```python
from build123d import *

# Parameters (mm, degrees)
F1_DEPTH = 6.35
F2_W     = 6.35
F2_H     = 6.35
F3_DEPTH = 6.351


with BuildPart() as f1:
    # F0 (on Right) → F1 (new body)
    with BuildSketch(Plane.YZ):
        Polygon((-38.1, 38.1), (-44.45, 38.1), (-44.45, 31.75), (-50.8, 31.75), (-50.8, 25.4), (-44.45, 25.4), (-44.45, 19.05), (-50.8, 19.05), (-50.8, 12.7), (-44.45, 12.7), (-44.45, 6.35), (-50.8, 6.35), (-50.8, 0), (-50.8, -6.35), (-44.45, -6.35), (-44.45, -12.7), (-50.8, -12.7), (-50.8, -19.05), (-44.45, -19.05), (-44.45, -25.4), (-50.8, -25.4), (-50.8, -31.75), (-44.45, -31.75), (-44.45, -38.1), (-38.1, -38.1), (-38.1, -31.75), (-31.75, -31.75), (-31.75, -38.1), (-25.4, -38.1), (-25.4, -31.75), (-19.05, -31.75), (-19.05, -38.1), (-12.7, -38.1), (-12.7, -31.75), (-6.35, -31.75), (-6.35, -38.1), (0, -38.1), (6.35, -38.1), (6.35, -31.75), (12.7, -31.75), (12.7, -38.1), (19.05, -38.1), (19.05, -31.75), (25.4, -31.75), (25.4, -38.1), (31.75, -38.1), (31.75, -31.75), (38.1, -31.75), (38.1, -38.1), (44.45, -38.1), (44.45, -31.75), (50.8, -31.75), (50.8, -25.4), (44.45, -25.4), (44.45, -19.05), (50.8, -19.05), (50.8, -12.7), (44.45, -12.7), (44.45, -6.35), (50.8, -6.35), (50.8, 0), (50.8, 6.35), (44.45, 6.35), (44.45, 12.7), (50.8, 12.7), (50.8, 19.05), (44.45, 19.05), (44.45, 25.4), (50.8, 25.4), (50.8, 31.75), (44.45, 31.75), (44.45, 38.1), (38.1, 38.1), (38.1, 31.75), (31.75, 31.75), (31.75, 38.1), (25.4, 38.1), (25.4, 31.75), (19.05, 31.75), (19.05, 38.1), (12.7, 38.1), (12.7, 31.75), (6.35, 31.75), (6.35, 38.1), (0, 38.1), (-6.35, 38.1), (-6.35, 31.75), (-12.7, 31.75), (-12.7, 38.1), (-19.05, 38.1), (-19.05, 31.75), (-25.4, 31.75), (-25.4, 38.1), (-31.75, 38.1), (-31.75, 31.75), (-38.1, 31.75), align=None)
    extrude(amount=F1_DEPTH)

    # F2 (on face) → F3 (cut, through all)
    with BuildSketch(Plane.YZ.offset(6.35)):
        with BuildLine():
            ThreePointArc((-15.875, -6.35), (-12.7, -7.6651280605), (-9.525, -6.35))
            Line((-9.525, -6.35), (-15.875, -6.35))
        make_face()
        Polygon((-15.875, -6.35), (-9.525, -6.35), (-9.525, -3.175), (-9.525, 0), (-15.875, 0), align=None)
        with BuildLine():
            Line((-9.525, -3.175), (-9.525, -6.35))
            ThreePointArc((-9.525, -6.35), (-8.5516625865, -4.893297618), (-8.2098719395, -3.175))
            ThreePointArc((-8.2098719395, -3.175), (-8.5516625865, -1.456702382), (-9.525, 0))
            Line((-9.525, 0), (-9.525, -3.175))
        make_face()
        with BuildLine():
            ThreePointArc((-15.875, 0), (-17.1901280605, -3.175), (-15.875, -6.35))
            Line((-15.875, -6.35), (-15.875, 0))
        make_face()
        with BuildLine():
            Line((-15.875, 0), (-9.525, 0))
            ThreePointArc((-9.525, 0), (-12.7, 1.3151280605), (-15.875, 0))
        make_face()
        with BuildLine():
            ThreePointArc((22.225, 0), (19.05, 1.3151280605), (15.875, 0))
            Line((15.875, 0), (22.225, 0))
        make_face()
        with Locations((19.05, -3.175)):
            Rectangle(F2_W, F2_H)
        with BuildLine():
            Line((15.875, -6.35), (15.875, 0))
            ThreePointArc((15.875, 0), (14.5598719395, -3.175), (15.875, -6.35))
        make_face()
        with BuildLine():
            ThreePointArc((23.5401280605, -3.175), (23.1983374135, -1.456702382), (22.225, 0))
            Line((22.225, 0), (22.225, -6.35))
            ThreePointArc((22.225, -6.35), (23.1983374135, -4.893297618), (23.5401280605, -3.175))
        make_face()
        with BuildLine():
            Line((22.225, -6.35), (15.875, -6.35))
            ThreePointArc((15.875, -6.35), (19.05, -7.6651280605), (22.225, -6.35))
        make_face()
    extrude(amount=-F3_DEPTH, mode=Mode.SUBTRACT)


solid = f1.part
```
Part model, mm, in its own coordinate system. A direction names the side the tool comes from. Give positions to 0.01 mm unless a question says otherwise; leave off trailing zeros. Order: outer loops, then holes, each group sorted by start corner. A loop starts at its lowest first (then second) coordinate and runs counter-clockwise, first axis right, second up. Notation, with made-up numbers: M 39.25,43.25 L 48.25,43.25 A19 ccw 48.25,47.25 Z; hole C 34.25,-11 d6. An arc over 180 degrees is marked long. Use a Markdown table: item, result. Add a question column.
(1) Saw through at A-A, the plane y = 35. Give the cut face in (x, z), and give its area (3 significant figures).
(2) 3-axis set-ups, long thin cutter, end or side, ignore diameter. For faces 5 (the face through (3, -48, -19.05)), 6 (the face through (3, -31.75, 35)), 7 (the face through (3, 48, -31.75)), 8 (the face through (3, 31.75, -35)): which of +Z, -Z, +X, -X, +Y, -Y reach the whole face in a straight line?
(3) Probe line 1 along Z through (x, y) = (3.5, 45.5); line 2 along Z through (x, y) = (6, -13); line 3 along Y through (x, z) = (1.75, -11.5). List the from-to ranges inside material, lowest first. Write a range as [from, to].
(4) Saw through at B-B, the plane x = 2. Give the number of separate pieces and of enclosed holes in the cut face, and give its area (3 significant figures).
(5) Drop flat-ended pins along their axis: P1, Ø3, axis at x = 4, z = 34, coming from the +Y side; P2, Ø3, axis at x = 4.5, z = -34.5, coming from the -Y side; P3, Ø1.9, axis at x = 3.5, y = -49, coming from the -Z side; P4, Ø2, axis at x = 5, y = 7, coming from the -Z side. Give the stop position or say it passes through.
(6) Saw through at C-C, the plane z = -21.5. Give the cut face in (x, y), and give its area (3 significant figures).
(7) Mould opens along Y. For faces 1 (the face through (3, -50.8, 0)), 2 (the face through (3, -25.4, 35)), 3 (the face through (3, 41, 38.1)), 4 (the face through (3, 35, 31.75)) say: +Y half, -Y half, draft (parallel to the pull), parting line (faces both ways), or undercut.
Answer key:
| question | item | result |
|---|---|---|
| 1 | outline | M 0,-31.75 L 6.35,-31.75 L 6.35,31.75 L 0,31.75 Z |
| 1 | area | 403 mm^2 |
| 2 | face 5 | +X, -X, -Y |
| 2 | face 6 | +Z, +X, -X |
| 2 | face 7 | -Z, +X, -X, +Y |
| 2 | face 8 | -Z, +X, -X |
| 3 | line 1 | [-31.75, -25.4], [-19.05, -12.7], [-6.35, 6.35], [12.7, 19.05], [25.4, 31.75] |
| 3 | line 2 | [-38.1, -7.66], [1.31, 38.1] |
| 3 | line 3 | [-44.45, 44.45] |
| 4 | separate pieces | 1 |
| 4 | enclosed holes | 2 |
| 4 | area | 6,650 mm^2 |
| 5 | P1 | y = 44.45 |
| 5 | P2 | y = -44.45 |
| 5 | P3 | z = -31.75 |
| 5 | P4 | z = -38.1 |
| 6 | outline | M 0,-44.45 L 6.35,-44.45 L 6.35,44.45 L 0,44.45 Z |
| 6 | area | 565 mm^2 |
| 7 | face 1 | -Y half |
| 7 | face 2 | undercut |
| 7 | face 3 | draft |
| 7 | face 4 | undercut |
